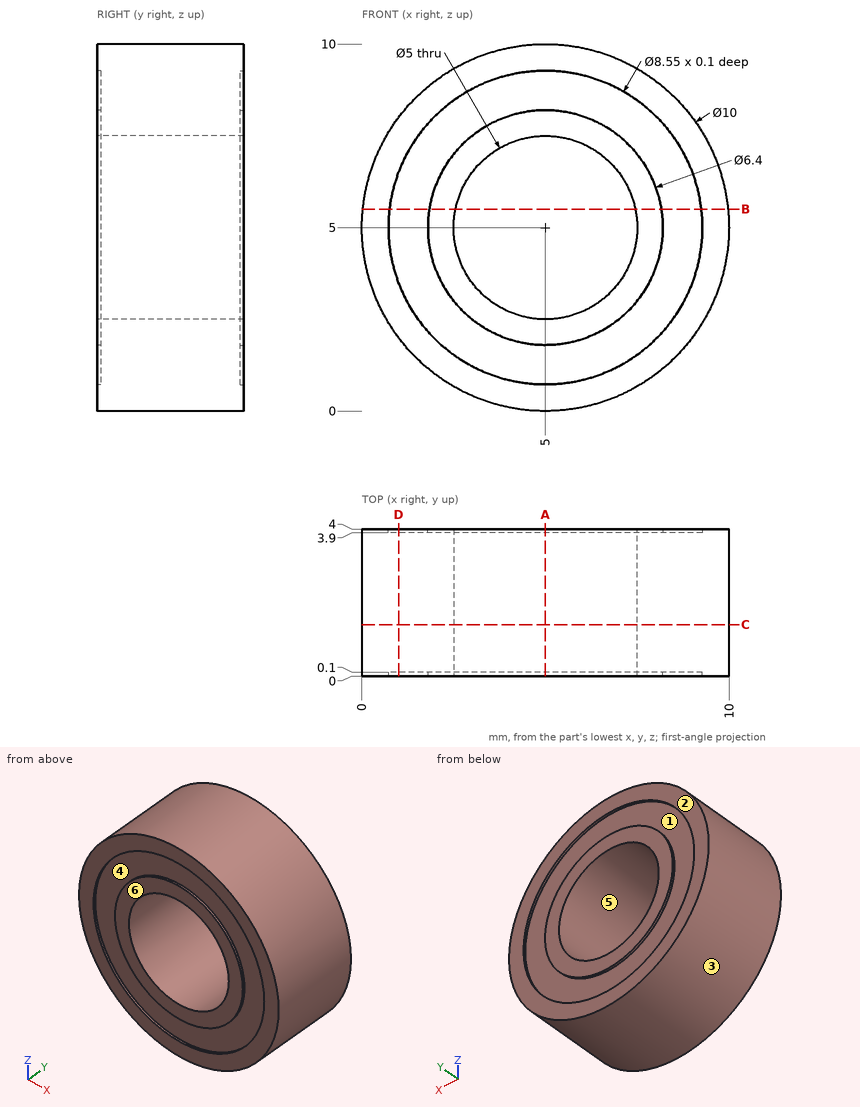
The drawing under review shows one solid part. Ordinate dimensions are in mm from its lowest x, y, z. A direction names the side the tool comes from. Give positions to 0.01 mm unless a question says otherwise; leave off trailing zeros. Write each loop counter-clockwise with the first axis right and the second up, starting at its lowest first coordinate (ties: lowest second). Pieces come first, ordered by that corner, then holes. Notation, with made-up numbers: M 31,-4 L 52,-4 A30 cw 52,33 Z; hole C -37,44.5 d11. An arc over 180 degrees is marked long. Write each question's results on one line, items separated by ' | '. Start each with the question number.
1. We need section B-B (z = 5.5). Write out the cut boundary in (x, y).
2. We need section D-D (x = 1). Write out the cut boundary in (y, z).
3. For the marked faces 1 and 2, list the 3-axis set-ups (+Z, -Z, +X, -X, +Y, -Y) from which the entire face can be reached by the end or side of a thin tool; tool diameter is ignored.
4. Insertion check: pin 1 Ø4 at (x, z) = (5, 5) entering from -Y. The pin has a flat end and moves straight along its axis. Give the tip position at first contact, or say it passes through.
5. We need section A-A (x = 5). Write out the cut boundary in (y, z) (3 decimals), and give its area (3 significant figures).
6. We need section C-C (y = 1.4). Write out the cut boundary in (x, z).
7. For probe 1 along Z at (x, y) = (5, 0.05) (3 decimals); probe 2 along Z at (x, y) = (5, 2.85), list the stretches that pass through material, from the lowest coordinate up. Write a range as [from, to].
8. Mouldability with a two-part tool opening along Z and no side actions: class the marked faces 3, 4, 5 and 6 as released by +Z, released by -Z, zero draft, split by the parting line, or undercut.
Results found:
1) outline: M 0.03,0 L 0.75,0 L 0.75,0.1 L 1.84,0.1 L 1.84,0 L 2.55,0 L 2.55,4 L 1.84,4 L 1.84,3.9 L 0.75,3.9 L 0.75,4 L 0.03,4 Z; M 7.45,0 L 8.16,0 L 8.16,0.1 L 9.25,0.1 L 9.25,0 L 9.97,0 L 9.97,4 L 9.25,4 L 9.25,3.9 L 8.16,3.9 L 8.16,4 L 7.45,4 Z
2) outline: M 0,2 L 4,2 L 4,3.49 L 3.9,3.49 L 3.9,6.51 L 4,6.51 L 4,8 L 0,8 L 0,6.51 L 0.1,6.51 L 0.1,3.49 L 0,3.49 Z
3) face 1: +Y | face 2: +Z, -Z, +X, -X, +Y
4) pin 1: passes through
5) outline: M 0,0 L 4,0 L 4,0.725 L 3.9,0.725 L 3.9,1.8 L 4,1.8 L 4,2.5 L 0,2.5 L 0,1.8 L 0.1,1.8 L 0.1,0.725 L 0,0.725 Z; M 0,7.5 L 4,7.5 L 4,8.2 L 3.9,8.2 L 3.9,9.275 L 4,9.275 L 4,10 L 0,10 L 0,9.275 L 0.1,9.275 L 0.1,8.2 L 0,8.2 Z | area: 19.6 mm^2
6) outline: C 5,5 d10; hole C 5,5 d5
7) probe 1: z = [0, 0.725], [1.8, 2.5], [7.5, 8.2], [9.275, 10] | probe 2: z = [0, 2.5], [7.5, 10]
8) face 3: split by the parting line | face 4: undercut | face 5: undercut | face 6: zero draft
